The listing builds one solid part. Answer for the finished solid, in the listing's coordinates (mm). A direction names the side the tool comes from. Round coordinates to 2 decimals unless told otherwise and drop trailing zeros. Order: outer loops, then holes, each group sorted by start corner. A loop starts at its lowest first (then second) coordinate and runs counter-clockwise, first axis right, second up. Notation, with made-up numbers: (14, 21) -> (35, 21) arc R28 cw to (35, 39) -> close; hole circle Ø6 at (70, -28). An arc over 180 degrees is marked (long way). Return JSON: item names as keys, results as strings. Group by question number.
(1) Consider line 1 (X direction, y = 4.7, z = -27); line 2 (X direction, y = 4.85, z = -63.5); line 3 (Z direction, x = -44, y = 2.05). Determine where each line is inside the solid, lowest interval first. Write a range as [from, to].
(2) The part is cut by section D-D (y = 1.5). Count the separate pieces of the cut face and the enclosed holes in it, plus the area to 3 significant figures.
(3) Which of the six approach directions +Z, -Z, +X, -X, +Y, -Y give full straight-line access (tool end or side, diameter ignored) to faces 1 (the face through (-30, 3, -148.781)), 2 (the face through (57.5, 3, -97)), 3 (the face through (63.966, 3, 45)), 4 (the face through (-61, 3, 0.219))?
(4) The part is cut by section A-A (x = -42). Determine the outline of the cut face in (y, z), plus the area to 3 significant figures.
(5) Each of these flat-tipped pins is pushed along its axis until it touches: pin 1 (3 mm diameter, centred on y = 3, z = 106, fed in from +X); pin 2 (3 mm diameter, centred on x = -60.5, y = 3.5, fed in from +Z); pin 3 (3 mm diameter, centred on y = 2.5, z = -144.5, fed in from +X). Where does it stop, or does it pass through?
(6) The part is cut by section C-C (x = -22.5). Determine the outline of the cut face in (y, z), plus the area to 3 significant figures.
(7) The part is cut by section B-B (z = 94.5). Determine the outline of the cut face in (x, y).
from build123d import *

# Parameters (mm, degrees)
SKETCH_1_R      = 30
SKETCH_1_W      = 25
SKETCH_1_H      = 67
EXTRUDE_1_DEPTH = 6


with BuildPart() as part:
    # Эскиз1 → Бобышка-Вытянуть1 (new body)
    with BuildSketch(Plane(origin=(0, 0, 0), x_dir=(1, 0, 0), z_dir=(0, 1, 0))):
        Polygon((-63.5, -90.219106224), (-63.5, -120.219106224), (-57.5, -120.219106224), (-57.5, -127.987103964), (-44.534331601, -127.987103964), (-14.534331601, -127.987103964), (15.172762814, -127.987103964), (45.172762814, -127.987103964), (57.756160079, -127.987103964), (57.965668399, -119.808299483), (63.965668399, -119.808299483), (63.965668399, -89.808299483), (57.965668399, -89.808299483), (57.965668399, -59.808299483), (63.965668399, -59.808299483), (63.965668399, -29.808299483), (57.965668399, -29.808299483), (57.965668399, 0.191700517), (64.611703668, 0.204499173), (64.557084704, 30.204449452), (58.557094649, 30.193525659), (58.502475685, 60.193475939), (64.331284091, 60.191395834), (64.331888746, 90.191395828), (57.5, 90.191533526), (57.5, 104.982806986), (63.5, 104.982806986), (63.5, 134.982806986), (57.5, 134.982806986), (57.5, 152.780893776), (-14.534331601, 152.780893776), (-57.5, 152.780893776), (-57.5, 134.982806986), (-63.5, 134.982806986), (-63.5, 104.982806986), (-57.5, 104.982806986), (-57.5, 89.780893776), (-63.5, 89.780893776), (-63.5, 59.780893776), (-63.034331601, 59.780893776), (-57.5, 59.780893776), (-57.5, 42.012896036), (-57.5, 29.780893776), (-63.5, 29.780893776), (-63.5, -0.219106224), (-63.034331601, -0.219106224), (-57.5, -0.219106224), (-57.5, -17.987103964), (-57.5, -30.219106224), (-63.5, -30.219106224), (-63.5, -60.219106224), (-63.034331601, -60.219106224), (-57.5, -60.219106224), (-57.5, -77.987103964), (-57.5, -90.219106224), align=None)
        with Locations(Location((21.965668399, -74.808299483, 0), (0, 0, 270))):
            Circle(SKETCH_1_R, mode=Mode.SUBTRACT)
        with Locations((-22.350212696, 43.691700517)):
            Rectangle(SKETCH_1_W, SKETCH_1_H, mode=Mode.SUBTRACT)
        Polygon((-14.534331601, 142.780893776), (-44.534331601, 142.780893776), (-44.534331601, 146.780893776), (-44.534331601, 148.780893776), (-14.534331601, 148.780893776), (-14.534331601, 146.780893776), align=None, mode=Mode.SUBTRACT)
        with Locations((22.649787304, 43.691700517)):
            Rectangle(SKETCH_1_W, SKETCH_1_H, mode=Mode.SUBTRACT)
        Polygon((45.172762814, 142.780893776), (15.172762814, 142.780893776), (15.172762814, 146.780893776), (15.172762814, 148.780893776), (45.172762814, 148.780893776), (45.172762814, 146.780893776), align=None, mode=Mode.SUBTRACT)
    extrude(amount=EXTRUDE_1_DEPTH)


solid = part.part
Answer below:
{
 "1": {"line 1": "x = [-63.5, -34.85], [-9.85, 10.15], [35.15, 64.56]", "line 2": "x = [-63.5, -34.85], [-9.85, 10.15], [35.15, 64.33]", "line 3": "z = [-152.78, -148.78], [-142.78, 127.99]"},
 "2": {"separate pieces": "1", "enclosed holes": "5", "area": "27,700 mm²"},
 "3": {"face 1": "+Y, -Y", "face 2": "+X, +Y, -Y", "face 3": "+Z, +X, +Y, -Y", "face 4": "-X, +Y, -Y"},
 "4": {"outline": "(0, -152.78) -> (6, -152.78) -> (6, -148.78) -> (0, -148.78) -> close; (0, -142.78) -> (6, -142.78) -> (6, 127.99) -> (0, 127.99) -> close", "area": "1,650 mm²"},
 "5": {"pin 1": "stops at x = 63.97", "pin 2": "stops at z = 120.22", "pin 3": "stops at x = 57.5"},
 "6": {"outline": "(0, -152.78) -> (6, -152.78) -> (6, -148.78) -> (0, -148.78) -> close; (0, -142.78) -> (6, -142.78) -> (6, -77.19) -> (0, -77.19) -> close; (0, -10.19) -> (6, -10.19) -> (6, 127.99) -> (0, 127.99) -> close", "area": "1,250 mm²"},
 "7": {"outline": "(-63.5, 0) -> (-0.67, 0) -> (-0.67, 6) -> (-63.5, 6) -> close; (44.6, 0) -> (63.97, 0) -> (63.97, 6) -> (44.6, 6) -> close"}
}
